Source: CAD feature listing. Evaluate the final solid. Frame: model axes, mm. A direction names the side the tool comes from. Give positions to 0.01 mm unless a question says otherwise; leave off trailing zeros. Order: outer loops, then holes, each group sorted by start corner. A loop starts at its lowest first (then second) coordinate and runs counter-clockwise, first axis right, second up.
```python
from build123d import *

# Parameters (mm, degrees)
SKIZZE1_W                       = 42.3
SKIZZE1_H                       = 42.3
AUFSATZ_LINEAR_AUSTRAGEN1_DEPTH = 40
FASE1_SIZE                      = 3.5
SCHNITT_LINEAR_AUSTRAGEN1_DEPTH = 15
FASE2_SIZE                      = 0.5
AUFSATZ_LINEAR_AUSTRAGEN2_DEPTH = 5
M3_GEWINDEBOHRUNG1_D            = 2.5
M3_GEWINDEBOHRUNG1_DEPTH        = 5
M3_GEWINDEBOHRUNG1_TIP          = 0.751075774
FASE3_SIZE                      = 1
SCHNITT_LINEAR_START            = -7
SCHNITT_LINEAR_AUSTRAGEN2_DEPTH = 26


with BuildPart() as part:
    # Skizze1 → Aufsatz-Linear austragen1 (new body)
    with BuildSketch(Plane.XY):
        Rectangle(SKIZZE1_W, SKIZZE1_H)
    extrude(amount=AUFSATZ_LINEAR_AUSTRAGEN1_DEPTH)

    # Skizze3 → Rotation1 (revolve)
    with BuildSketch(Plane(origin=(0, 0, 0), x_dir=(0, 0, -1), z_dir=(1, 0, 0))):
        Polygon((-40, 18), (-67.3, 18), (-67.3, 11), (-68.3, 11), (-68.3, 4), (-87.3, 4), (-87.3, 0), (-40, 0), align=None)
    revolve(axis=Axis((0, 0, 0), (0, 0, 1)))

    # Fase1
    fase1_edges = [part.edges().sort_by_distance(p)[0] for p in [
        (-21.15, 21.15, 20),
        (21.15, 21.15, 20),
        (21.15, -21.15, 20),
        (-21.15, -21.15, 20),
    ]]
    chamfer(fase1_edges, length=FASE1_SIZE)

    # Skizze4 → Schnitt-Linear austragen1 (cut)
    with BuildSketch(Plane.XY.offset(87.3)):
        with BuildLine():
            Line((-2.645751311, 3), (2.645751311, 3))
            ThreePointArc((2.645751311, 3), (0, 4), (-2.645751311, 3))
        make_face()
    extrude(amount=-SCHNITT_LINEAR_AUSTRAGEN1_DEPTH, mode=Mode.SUBTRACT)

    # Fase2
    fase2_edges = [part.edges().sort_by_distance(p)[0] for p in [
        (0, -4, 87.3),
    ]]
    chamfer(fase2_edges, length=FASE2_SIZE)

    # Skizze5 → Aufsatz-Linear austragen2 (add)
    with BuildSketch(Plane.XY.offset(40)):
        Polygon((20.15, 17.235786438), (17.235786438, 20.15), (-17.235786438, 20.15), (-20.15, 17.235786438), (-20.15, -17.235786438), (-17.235786438, -20.15), (17.235786438, -20.15), (20.15, -17.235786438), align=None)
    extrude(amount=AUFSATZ_LINEAR_AUSTRAGEN2_DEPTH)

    # M3 Gewindebohrung1
    with Locations(Plane.XY.offset(67.3)):
        with Locations((9.899494937, 9.899494937), (-9.899494937, 9.899494937), (-9.899494937, -9.899494937), (9.899494937, -9.899494937)):
            Hole(M3_GEWINDEBOHRUNG1_D / 2, depth=M3_GEWINDEBOHRUNG1_DEPTH)
            with Locations((0, 0, -(M3_GEWINDEBOHRUNG1_DEPTH + M3_GEWINDEBOHRUNG1_TIP / 2))):  # 118° drill point
                Cone(0, M3_GEWINDEBOHRUNG1_D / 2, M3_GEWINDEBOHRUNG1_TIP, mode=Mode.SUBTRACT)

    # Fase3
    fase3_edges = [part.edges().sort_by_distance(p)[0] for p in [
        (0, -18, 67.3),
    ]]
    chamfer(fase3_edges, length=FASE3_SIZE)

    # Skizze8 → Schnitt-Linear austragen2 (cut)
    with BuildSketch(Plane(origin=(0, 0, 0), x_dir=(-1, 0, 0), z_dir=(0, 0, -1)).offset(SCHNITT_LINEAR_START)):
        Polygon((17.65, 21.15), (-17.65, 21.15), (-21.15, 17.65), (-21.15, -17.65), (-17.65, -21.15), (17.65, -21.15), (21.15, -17.65), (21.15, 17.65), align=None)
        Polygon((17.442893219, 20.65), (-17.442893219, 20.65), (-20.65, 17.442893219), (-20.65, -17.442893219), (-17.442893219, -20.65), (17.442893219, -20.65), (20.65, -17.442893219), (20.65, 17.442893219), align=None, mode=Mode.SUBTRACT)
    extrude(amount=-SCHNITT_LINEAR_AUSTRAGEN2_DEPTH, mode=Mode.SUBTRACT)


solid = part.part
```
1) Section query D-D, the plane z = 77. Return the cut outline in (x, y).
Report:
outline: (-2.65, 3) arc R4 ccw (long way) to (2.65, 3) - close
2) Pin query (flat end, axial travel): pin 1 (8 mm diameter, centred on y = -1.5, z = 21, fed in from -X); pin 2 (5 mm diameter, centred on x = -6.5, y = 7, fed in from +Z); pin 3 (2 mm diameter, centred on x = 12, y = -2.5, fed in from +Z). Return the tip coordinate at first contact, or that it passes through.
Report:
pin 1: stops at x = -20.65
pin 2: stops at z = 68.3
pin 3: stops at z = 67.3
3) Reachability of faces 1 (the flat face through (-18.713, -18.672, 42.465)), 2 (the flat face through (0, 20.65, 20)), 3 (the cylindrical face through (10.74, -2.38, 67.81)), 4 (the flat face through (19.069, -19.024, 19.818)), 5 (the flat face through (0, -20.15, 42)) from +Z, -Z, +X, -X, +Y, -Y: full face, straight path, thin tool, end or side. Return the list, or none.
Report:
face 1: +Z, -X, -Y
face 2: +X, -X, +Y
face 3: +Z
face 4: +X, -Y
face 5: +Z, +X, -X, -Y
4) Material intervals for L1, parallel to Y at x = 11, z = 64; L2, parallel to Z at x = 15, y = 6.5; L3, parallel to Y at x = -9.5, z = 41.5, sorted ascending.
Report:
L1: y = -14.25 to -10.49, -9.31 to 9.31, 10.49 to 14.25
L2: z = 0 to 67.3
L3: y = -20.15 to 20.15
5) Section query B-B, the plane z = 43.5. Return the cut outline in (x, y), and give its area (3 significant figures).
Report:
outline: (-20.15, -17.24) - (-17.24, -20.15) - (17.24, -20.15) - (20.15, -17.24) - (20.15, 17.24) - (17.24, 20.15) - (-17.24, 20.15) - (-20.15, 17.24) - close
area: 1,610 mm2
6) Draft query along X for faces 6 (the flat face through (19.4, 19.4, 36.5)), 7 (the conical face through (-9.95, -10.11, 61.68)), 8 (the flat face through (-21.15, 0, 36)). Return one class per face: +X half, -X half, draft (parallel to the pull), parting line (faces both ways), or undercut.
Report:
face 6: +X half
face 7: undercut
face 8: -X half
